Input: dimensioned drawing with shaded views. Units: mm. Origin: part minimum x, y, z. Give positions to 0.01 mm unless a question says otherwise; leave off trailing zeros. Order: outer loops, then holes, each group sorted by start corner. A loop starts at its lowest first (then second) coordinate and runs counter-clockwise, first axis right, second up. Notation, with made-up numbers: M -22.75,79 L 25.25,79 A16 cw 25.25,94 Z; hole C 82.5,77 d3. An arc over 180 degrees is marked long. Answer in a Markdown table with one row per item. Add a question column.
(1) Section query C-C, the plane x = 105.5. Return loops of the section in (y, z), plus the area to 3 significant figures.
(2) Section query D-D, the plane x = 20. Return loops of the section in (y, z), plus the area to 3 significant figures.
(3) Section query A-A, the plane x = 211. Return loops of the section in (y, z).
(4) Section query B-B, the plane x = 278.5. Return loops of the section in (y, z), plus the area to 3 significant figures.
(5) Material intervals for line 1 along Y through (x, z) = (26, 2) (1 decimal); line 2 along X through (y, z) = (146.5, 5.75) (1 decimal); line 3 along Y through (x, z) = (213, 5) (1 decimal), sorted ascending.
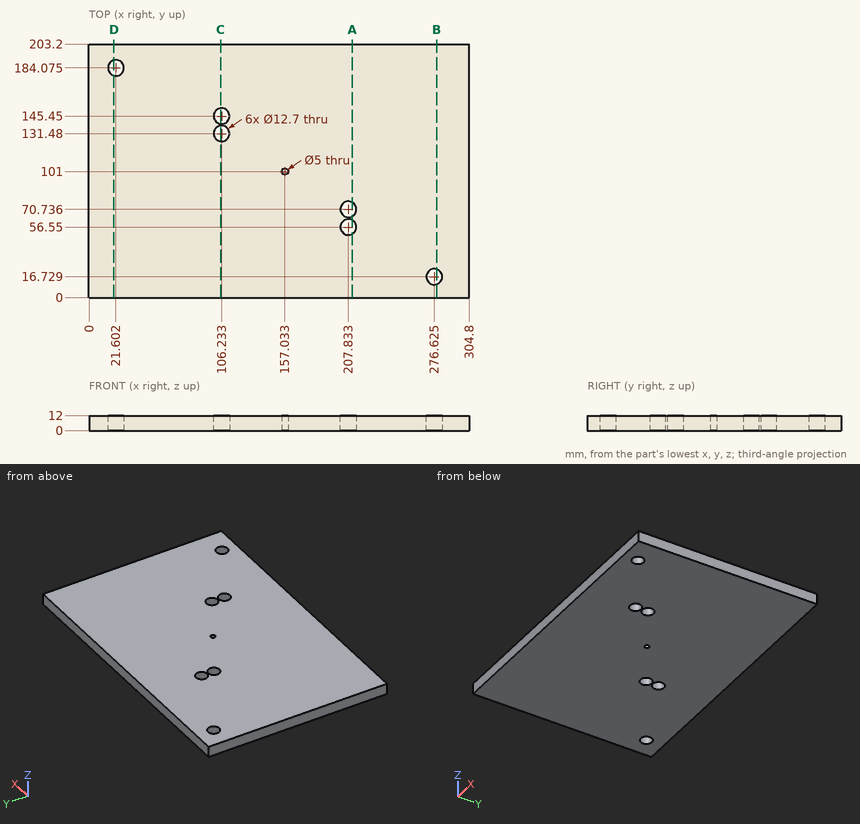
Values follow:
| question | item | result |
|---|---|---|
| 1 | outline | M 0,0 L 125.17,0 L 125.17,12 L 0,12 Z; M 137.79,0 L 139.14,0 L 139.14,12 L 137.79,12 Z; M 151.76,0 L 203.2,0 L 203.2,12 L 151.76,12 Z |
| 1 | area | 2,140 mm² |
| 2 | outline | M 0,0 L 177.93,0 L 177.93,12 L 0,12 Z; M 190.22,0 L 203.2,0 L 203.2,12 L 190.22,12 Z |
| 2 | area | 2,290 mm² |
| 3 | outline | M 0,0 L 51.05,0 L 51.05,12 L 0,12 Z; M 62.05,0 L 65.23,0 L 65.23,12 L 62.05,12 Z; M 76.24,0 L 203.2,0 L 203.2,12 L 76.24,12 Z |
| 4 | outline | M 0,0 L 10.66,0 L 10.66,12 L 0,12 Z; M 22.8,0 L 203.2,0 L 203.2,12 L 22.8,12 Z |
| 4 | area | 2,290 mm² |
| 5 | line 1 | y = 0 to 179.5, 188.7 to 203.2 |
| 5 | line 2 | x = 0 to 100, 112.5 to 304.8 |
| 5 | line 3 | y = 0 to 52.9, 60.2 to 67, 74.4 to 203.2 |
